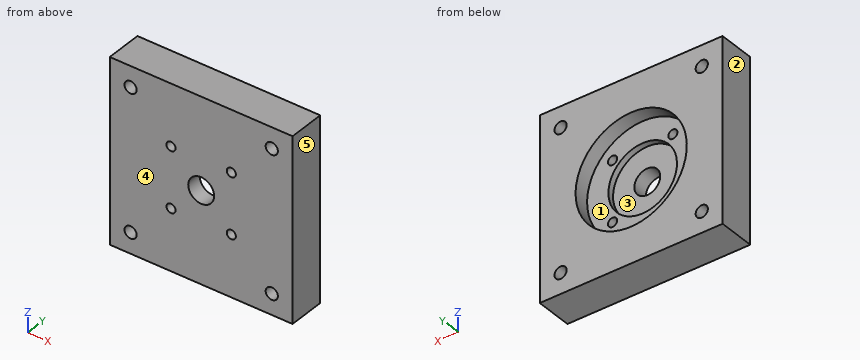
from build123d import *

# Parameters (mm, degrees)
SKETCH_1_W      = 60
SKETCH_1_H      = 60
SKETCH_1_R      = 1.5
SKETCH_1_R_2    = 2
SKETCH_1_R_3    = 4.25
EXTRUDE_1_DEPTH = 5
SKETCH_2_W      = 60
SKETCH_2_H      = 60
SKETCH_2_R      = 2
SKETCH_2_R_2    = 1.5
SKETCH_2_R_3    = 11.25
EXTRUDE_2_DEPTH = 2
SKETCH_3_W      = 60
SKETCH_3_H      = 60
SKETCH_3_R      = 18.25
SKETCH_3_R_2    = 2
EXTRUDE_3_DEPTH = 5


with BuildPart() as part:
    # 草图1 → 凸台-拉伸1 (new body)
    with BuildSketch(Plane(origin=(0, 0, 0), x_dir=(1, 0, 0), z_dir=(0, 1, 0))):
        Rectangle(SKETCH_1_W, SKETCH_1_H)
        with Locations(Location((-9.899494937, 9.899494937, 0), (0, 0, 270))):
            Circle(SKETCH_1_R, mode=Mode.SUBTRACT)
        with Locations(Location((9.899494937, 9.899494937, 0), (0, 0, 270))):
            Circle(SKETCH_1_R, mode=Mode.SUBTRACT)
        with Locations(Location((9.899494937, -9.899494937, 0), (0, 0, 270))):
            Circle(SKETCH_1_R, mode=Mode.SUBTRACT)
        with Locations(Location((-9.899494937, -9.899494937, 0), (0, 0, 270))):
            Circle(SKETCH_1_R, mode=Mode.SUBTRACT)
        with Locations(Location((-23.171320344, 23.171320344, 0), (0, 0, 270))):
            Circle(SKETCH_1_R_2, mode=Mode.SUBTRACT)
        with Locations(Location((23.171320344, 23.171320344, 0), (0, 0, 270))):
            Circle(SKETCH_1_R_2, mode=Mode.SUBTRACT)
        with Locations(Location((-23.171320344, -23.171320344, 0), (0, 0, 270))):
            Circle(SKETCH_1_R_2, mode=Mode.SUBTRACT)
        with Locations(Location((23.171320344, -23.171320344, 0), (0, 0, 270))):
            Circle(SKETCH_1_R_2, mode=Mode.SUBTRACT)
        with Locations(Location((0, 0, 0), (0, 0, 270))):
            Circle(SKETCH_1_R_3, mode=Mode.SUBTRACT)
    extrude(amount=EXTRUDE_1_DEPTH)

    # 草图2 → 凸台-拉伸2 (add)
    with BuildSketch(Plane(origin=(0, 5, 0), x_dir=(1, 0, 0), z_dir=(0, 1, 0))):
        Rectangle(SKETCH_2_W, SKETCH_2_H)
        with Locations(Location((-23.171320344, -23.171320344, 0), (0, 0, 270))):
            Circle(SKETCH_2_R, mode=Mode.SUBTRACT)
        with Locations(Location((23.171320344, 23.171320344, 0), (0, 0, 270))):
            Circle(SKETCH_2_R, mode=Mode.SUBTRACT)
        with Locations(Location((23.171320344, -23.171320344, 0), (0, 0, 270))):
            Circle(SKETCH_2_R, mode=Mode.SUBTRACT)
        with Locations(Location((-23.171320344, 23.171320344, 0), (0, 0, 270))):
            Circle(SKETCH_2_R, mode=Mode.SUBTRACT)
        with Locations(Location((-9.899494937, -9.899494937, 0), (0, 0, 270))):
            Circle(SKETCH_2_R_2, mode=Mode.SUBTRACT)
        with Locations(Location((9.899494937, -9.899494937, 0), (0, 0, 270))):
            Circle(SKETCH_2_R_2, mode=Mode.SUBTRACT)
        with Locations(Location((9.899494937, 9.899494937, 0), (0, 0, 270))):
            Circle(SKETCH_2_R_2, mode=Mode.SUBTRACT)
        with Locations(Location((-9.899494937, 9.899494937, 0), (0, 0, 270))):
            Circle(SKETCH_2_R_2, mode=Mode.SUBTRACT)
        with Locations(Location((0, 0, 0), (0, 0, 270))):
            Circle(SKETCH_2_R_3, mode=Mode.SUBTRACT)
    extrude(amount=EXTRUDE_2_DEPTH)

    # 草图3 → 凸台-拉伸3 (add)
    with BuildSketch(Plane(origin=(0, 7, 0), x_dir=(1, 0, 0), z_dir=(0, 1, 0))):
        Rectangle(SKETCH_3_W, SKETCH_3_H)
        with Locations(Location((0, 0, 0), (0, 0, 270))):
            Circle(SKETCH_3_R, mode=Mode.SUBTRACT)
        with Locations(Location((-23.171320344, -23.171320344, 0), (0, 0, 270))):
            Circle(SKETCH_3_R_2, mode=Mode.SUBTRACT)
        with Locations(Location((23.171320344, 23.171320344, 0), (0, 0, 270))):
            Circle(SKETCH_3_R_2, mode=Mode.SUBTRACT)
        with Locations(Location((23.171320344, -23.171320344, 0), (0, 0, 270))):
            Circle(SKETCH_3_R_2, mode=Mode.SUBTRACT)
        with Locations(Location((-23.171320344, 23.171320344, 0), (0, 0, 270))):
            Circle(SKETCH_3_R_2, mode=Mode.SUBTRACT)
    extrude(amount=EXTRUDE_3_DEPTH)


solid = part.part
Source: CAD feature listing. Evaluate the final solid. Frame: model axes, mm. Face numbers are marked on the shaded views. A direction names the side the tool comes from. Coordinates: 2 decimals unless noted, no trailing zeros. Order: outer loops, then holes, each group sorted by start corner. A loop starts at its lowest first (then second) coordinate and runs counter-clockwise, first axis right, second up. Notation, with made-up numbers: M 35,56 L 46,56 A11 ccw 46,66 Z; hole C -13,-23 d10. An arc over 180 degrees is marked long. Write each question's results on one line, items separated by ' | '. Start each with the question number.
Item 1: Cut plane D-D (x = -7). Return loops of the section in (y, z), and give its area (3 significant figures).
Item 2: Set-up query: the marked faces 1 and 2. Return all of +Z, -Z, +X, -X, +Y, -Y with unobstructed straight access to the full face (end or side cutting, diameter ignored); none if empty.
Item 3: Cut plane A-A (x = 0). Return loops of the section in (y, z), and give its area (3 significant figures).
Item 4: First-contact query: pin 1 Ø7 at (x, z) = (3, -4.5) entering from +Y; pin 2 Ø2.5 at (x, z) = (-9.9, -9.9) entering from +Y. Flat tips, straight axial feed; report the tip coordinate or a pass-through.
Item 5: Cut plane C-C (y = 2.25). Count the separate pieces of the cut face and the enclosed holes in it, and give its area (3 significant figures).
Item 6: Line query: probe 1 along X at (y, z) = (7.75, -24); probe 2 along Z at (x, y) = (23.5, 6.25); probe 3 along X at (y, z) = (10, 0). Output: solid intervals per line, ascending.
Item 7: Draft query along X for the marked faces 3, 4 and 5. Return one class per face: pulls with the +X half, pulls with the -X half, needs draft (parallel to the pull), parting line crosses it, or undercut.
Item 8: Cut plane B-B (z = 0). Return loops of the section in (x, y), and give its area (3 significant figures).
Checked values:
1) outline: M 0,-30 L 12,-30 L 12,-16.85 L 7,-16.85 L 7,-8.81 L 5,-8.81 L 5,8.81 L 7,8.81 L 7,16.85 L 12,16.85 L 12,30 L 0,30 Z | area: 516 mm2
2) face 1: +Y | face 2: +Z, -Z, -X, +Y, -Y
3) outline: M 0,-30 L 12,-30 L 12,-18.25 L 7,-18.25 L 7,-11.25 L 5,-11.25 L 5,-4.25 L 0,-4.25 Z; M 0,4.25 L 5,4.25 L 5,11.25 L 7,11.25 L 7,18.25 L 12,18.25 L 12,30 L 0,30 Z | area: 450 mm2
4) pin 1: stops at y = 5 | pin 2: passes through
5) separate pieces: 1 | enclosed holes: 9 | area: 3,460 mm2
6) probe 1: x = -30 to -24.99, -21.35 to 21.35, 24.99 to 30 | probe 2: z = -30 to -25.14, -21.2 to 21.2, 25.14 to 30 | probe 3: x = -30 to -18.25, 18.25 to 30
7) face 3: undercut | face 4: needs draft | face 5: pulls with the +X half
8) outline: M -30,0 L -4.25,0 L -4.25,5 L -11.25,5 L -11.25,7 L -18.25,7 L -18.25,12 L -30,12 Z; M 4.25,0 L 30,0 L 30,12 L 18.25,12 L 18.25,7 L 11.25,7 L 11.25,5 L 4.25,5 Z | area: 450 mm2
